from build123d import *

# Parameters (mm, degrees)
SKETCH016_W     = 96
SKETCH016_H     = 70
PAD003_DEPTH    = 3
SKETCH017_W     = 6.3
SKETCH017_H     = 6.3
PAD004_DEPTH    = 2.7
SKETCH018_R     = 1.7
POCKET013_DEPTH = 5.701
SKETCH019_W     = 79.4
SKETCH019_H     = 2
SKETCH019_W_2   = 2
SKETCH019_H_2   = 53.8
PAD005_DEPTH    = 1
SKETCH020_W     = 9
SKETCH020_H     = 1.8
PAD006_DEPTH    = 4.3
SKETCH021_W     = 9
SKETCH021_H     = 0.3
POCKET014_DEPTH = 3.3
SKETCH022_W     = 2
SKETCH022_H     = 5.4
PAD007_DEPTH    = 1
SKETCH023_W     = 1.7
SKETCH023_H     = 5.4
PAD008_DEPTH    = 10.6
SKETCH024_R     = 3
POCKET015_DEPTH = 96.001
SKETCH025_W     = 1.7
SKETCH025_H     = 5.4
PAD009_DEPTH    = 10.6
SKETCH026_R     = 3
POCKET016_DEPTH = 96.001
FILLET004_R     = 1
FILLET005_R     = 1
CHAMFER001_SIZE = 1.4


with BuildPart() as part:
    # Sketch016 → Pad003 (new body)
    with BuildSketch(Plane.XY.offset(22.8)):
        Rectangle(SKETCH016_W, SKETCH016_H)
    extrude(amount=PAD003_DEPTH)

    # Sketch017 (on Face5 of Pad003) → Pad004 (join)
    with BuildSketch(Plane(origin=(0, 0, 22.8), x_dir=(1, 0, 0), z_dir=(0, 0, -1))):
        with Locations((-42.85, 30.05)):
            Rectangle(SKETCH017_W, SKETCH017_H)
        with Locations((42.85, 30.05)):
            Rectangle(SKETCH017_W, SKETCH017_H)
        with Locations((42.85, -30.05)):
            Rectangle(SKETCH017_W, SKETCH017_H)
        with Locations((-42.85, -30.05)):
            Rectangle(SKETCH017_W, SKETCH017_H)
    extrude(amount=PAD004_DEPTH)

    # Sketch018 (on Face5 of Pad004) → Pocket013 (cut, through all)
    with BuildSketch(Plane.XY.offset(25.8)):
        with Locations((-43, 30.2)):
            Circle(SKETCH018_R)
        with Locations((43, 30.2)):
            Circle(SKETCH018_R)
        with Locations((43, -30.2)):
            Circle(SKETCH018_R)
        with Locations((-43, -30.2)):
            Circle(SKETCH018_R)
    extrude(amount=-POCKET013_DEPTH, mode=Mode.SUBTRACT)

    # Sketch019 (on Face4 of Pocket013) → Pad005 (join)
    with BuildSketch(Plane(origin=(0, 0, 22.8), x_dir=(1, 0, 0), z_dir=(0, 0, -1))):
        with Locations((0, -32.2)):
            Rectangle(SKETCH019_W, SKETCH019_H)
        with Locations((-45, 0)):
            Rectangle(SKETCH019_W_2, SKETCH019_H_2)
        with Locations((0, 32.2)):
            Rectangle(SKETCH019_W, SKETCH019_H)
        with Locations((45, 0)):
            Rectangle(SKETCH019_W_2, SKETCH019_H_2)
    extrude(amount=PAD005_DEPTH)

    # Sketch020 (on Face4 of Pad005) → Pad006 (join)
    with BuildSketch(Plane(origin=(0, 0, 22.8), x_dir=(1, 0, 0), z_dir=(0, 0, -1))):
        with Locations((17.1, -34.1)):
            Rectangle(SKETCH020_W, SKETCH020_H)
    extrude(amount=PAD006_DEPTH)

    # Sketch021 (on Face23 of Pad006) → Pocket014 (cut)
    with BuildSketch(Plane(origin=(0, 0, 18.5), x_dir=(1, 0, 0), z_dir=(0, 0, -1))):
        with Locations((17.1, -33.35)):
            Rectangle(SKETCH021_W, SKETCH021_H)
    extrude(amount=-POCKET014_DEPTH, mode=Mode.SUBTRACT)

    # Sketch022 (on Face4 of Pocket014) → Pad007 (join)
    with BuildSketch(Plane(origin=(0, 0, 22.8), x_dir=(1, 0, 0), z_dir=(0, 0, -1))):
        with Locations((-47, 9.5)):
            Rectangle(SKETCH022_W, SKETCH022_H)
        with Locations((-47, -9.5)):
            Rectangle(SKETCH022_W, SKETCH022_H)
    extrude(amount=PAD007_DEPTH)

    # Sketch023 (on Face39 of Pad007) → Pad008 (join)
    with BuildSketch(Plane(origin=(0, 0, 21.8), x_dir=(1, 0, 0), z_dir=(0, 0, -1))):
        with Locations((-47.15, -9.5)):
            Rectangle(SKETCH023_W, SKETCH023_H)
    extrude(amount=PAD008_DEPTH)

    # Sketch024 (on Face39 of Pad008) → Pocket015 (cut, through all)
    with BuildSketch(Plane(origin=(-48, 0, 0), x_dir=(0, -1, 0), z_dir=(-1, 0, 0))):
        with Locations((-9.5, 11.2)):
            Circle(SKETCH024_R)
    extrude(amount=-POCKET015_DEPTH, mode=Mode.SUBTRACT)

    # Sketch025 (on Face36 of Pocket015) → Pad009 (join)
    with BuildSketch(Plane(origin=(0, 0, 21.8), x_dir=(1, 0, 0), z_dir=(0, 0, -1))):
        with Locations((-47.15, 9.5)):
            Rectangle(SKETCH025_W, SKETCH025_H)
    extrude(amount=PAD009_DEPTH)

    # Sketch026 (on Face36 of Pad009) → Pocket016 (cut, through all)
    with BuildSketch(Plane(origin=(-48, 0, 0), x_dir=(0, -1, 0), z_dir=(-1, 0, 0))):
        with Locations((9.5, 11.2)):
            Circle(SKETCH026_R)
    extrude(amount=-POCKET016_DEPTH, mode=Mode.SUBTRACT)

    # Fillet004
    fillet004_edges = [part.edges().sort_by_distance(p)[0] for p in [
        (-39.7, -26.9, 21.45),
        (39.7, -26.9, 21.45),
        (39.7, 26.9, 21.45),
        (-39.7, 26.9, 21.45),
    ]]
    fillet(fillet004_edges, radius=FILLET004_R)

    # Fillet005
    fillet005_edges = [part.edges().sort_by_distance(p)[0] for p in [
        (-48, 35, 24.3),
        (-48, -35, 24.3),
        (48, -35, 24.3),
        (48, 35, 24.3),
    ]]
    fillet(fillet005_edges, radius=FILLET005_R)

    # Chamfer001
    chamfer001_edges = [part.edges().sort_by_distance(p)[0] for p in [
        (41.3, -30.2, 25.8),
        (-44.7, -30.2, 25.8),
        (41.3, 30.2, 25.8),
        (-44.7, 30.2, 25.8),
    ]]
    chamfer(chamfer001_edges, length=CHAMFER001_SIZE)


solid = part.part
Here's how the part is built. I have some questions about the finished solid (model axes, mm). A direction names the side the tool comes from. Coordinates: 2 decimals unless noted, no trailing zeros. Order: outer loops, then holes, each group sorted by start corner. A loop starts at its lowest first (then second) coordinate and runs counter-clockwise, first axis right, second up. Notation, with made-up numbers: M 40.5,32.5 L 87.5,32.5 A32 cw 87.5,63.5 Z; hole C -12,-12 d6. An arc over 180 degrees is marked long. Answer as CSV lines item,"result".
Item 1: Imagine slicing it at D-D on x = -3. Write out the boundary of the cut face in (y, z).
Results found:
outline,"M -35,22.8 L -33.2,22.8 L -33.2,21.8 L -31.2,21.8 L -31.2,22.8 L 31.2,22.8 L 31.2,21.8 L 33.2,21.8 L 33.2,22.8 L 35,22.8 L 35,25.8 L -35,25.8 Z"
Item 2: If I drill on line 1 (Y direction, x = -43, z = 21.15); line 2 (Y direction, x = 43, z = 23.3); line 3 (Z direction, x = -34.5, y = 29.5), over which ranges is the centre line in solid material (lowest first)?
Results found:
line 1,"-33.2 to -31.9, -28.5 to -26.9, 26.9 to 28.5, 31.9 to 33.2"
line 2,"-35 to -31.9, -28.5 to 28.5, 31.9 to 35"
line 3,"22.8 to 25.8"
Item 3: We'd pull the mould along Y, two halves only. Please class faces 4 (the face through (-47, 6.8, 18)), 5 (the face through (17, 33.5, 20)), 6 (the face through (-41, 29, 20.1)), 7 (the face through (45, 0, 21.8)): +Y half, -Y half, draft (parallel to the pull), parting line (faces both ways), or undercut.
Results found:
face 4,"undercut"
face 5,"-Y half"
face 6,"draft"
face 7,"undercut"
Item 4: Imagine slicing it at C-C on z = 17.5. Write out the boundary of the cut face in (x, y).
Results found:
outline,"M -48,-12.2 L -46.3,-12.2 L -46.3,-6.8 L -48,-6.8 Z; M -48,6.8 L -46.3,6.8 L -46.3,12.2 L -48,12.2 Z"
Item 5: Imagine slicing it at B-B on y = -30.2. Write out the boundary of the cut face in (x, z), plus the area to 3 significant figures.
Results found:
outline,"M -48,22.8 L -46,22.8 L -46,20.1 L -44.7,20.1 L -44.7,24.4 L -46.1,25.8 L -48,25.8 Z; M -41.3,20.1 L -39.7,20.1 L -39.7,22.8 L 39.7,22.8 L 39.7,20.1 L 41.3,20.1 L 41.3,24.4 L 39.9,25.8 L -39.9,25.8 L -41.3,24.4 Z; M 44.7,20.1 L 46,20.1 L 46,22.8 L 48,22.8 L 48,25.8 L 46.1,25.8 L 44.7,24.4 Z"
area,"279 mm2"
Item 6: Imagine slicing it at A-A on x = -43. Write out the boundary of the cut face in (y, z), plus the area to 3 significant figures.
Results found:
outline,"M -35,22.8 L -33.2,22.8 L -33.2,20.1 L -31.9,20.1 L -31.9,24.4 L -33.3,25.8 L -35,25.8 Z; M -28.5,20.1 L -26.9,20.1 L -26.9,22.8 L 26.9,22.8 L 26.9,20.1 L 28.5,20.1 L 28.5,24.4 L 27.1,25.8 L -27.1,25.8 L -28.5,24.4 Z; M 31.9,20.1 L 33.2,20.1 L 33.2,22.8 L 35,22.8 L 35,25.8 L 33.3,25.8 L 31.9,24.4 Z"
area,"201 mm2"
Item 7: For pin 1 (3 mm diameter, centred on x = 36, y = 20.5, fed in from -Z); pin 2 (3 mm diameter, centred on x = -42.5, z = 22, fed in from -Y); pin 3 (0.6 mm diameter, centred on x = -8.5, y = -32, fed in from -Z); pin 4 (0.8 mm diameter, centred on y = -31, z = 22, fed in from -X), each with a flat end and sliding along its axis, tell me the tip position at first contact or that it passes through.
Results found:
pin 1,"z = 22.8"
pin 2,"y = -35"
pin 3,"z = 21.8"
pin 4,"x = -46"
Item 8: On a 3-axis mill with a long thin cutter (end or side, diameter ignored), from which of +Z, -Z, +X, -X, +Y, -Y can I reach the whole of each face in a straight line? I mean faces 1 (the face through (-39.7, -31, 21)), 2 (the face through (-24, 33.2, 22)), 3 (the face through (-1, 32, 21.8)). Say none if no direction works.
Results found:
face 1,"-Z"
face 2,"-Z, -X, +Y"
face 3,"-Z, -Y"
